from build123d import *

# Parameters (mm, degrees)
BOSS_EXTRUDE1_DEPTH      = 266.7
BOSS_EXTRUDE1_DEPTH_BACK = 266.7
SKETCH3_W                = 25.4
SKETCH3_H                = 25.4
SKETCH3_W_2              = 19.05
SKETCH3_H_2              = 19.05
SKETCH4_R                = 9.525
CUT_EXTRUDE1_DEPTH       = 25.4
SKETCH5_R                = 9.525
CUT_EXTRUDE2_DEPTH       = 3.175
F_10_CLEARANCE_HOLE1_D   = 4.9784
F_10_CLEARANCE_HOLE2_D   = 4.9784


with BuildPart() as part:
    # Sketch3 → Boss-Extrude1 (new, two sides: drawn at the far end of the back side and taken through both)
    with BuildSketch(Plane.XY.offset(-BOSS_EXTRUDE1_DEPTH_BACK)):
        Rectangle(SKETCH3_W, SKETCH3_H)
        Rectangle(SKETCH3_W_2, SKETCH3_H_2, mode=Mode.SUBTRACT)
    extrude(amount=BOSS_EXTRUDE1_DEPTH + BOSS_EXTRUDE1_DEPTH_BACK)

    # Sketch4 → Cut-Extrude1 (cut)
    with BuildSketch(Plane(origin=(0, 12.7, 0), x_dir=(1, 0, 0), z_dir=(0, 1, 0))):
        with Locations(Location((0, 212.725, 0), (0, 0, 180))):
            Circle(SKETCH4_R)
        Polygon((-12.7, 225.013453558), (-12.7, 266.7), (12.7, 266.7), (12.7, 252.73), (-3.69434815, 252.73), align=None)
    extrude(amount=-CUT_EXTRUDE1_DEPTH, mode=Mode.SUBTRACT)

    # Sketch5 → Cut-Extrude2 (cut)
    with BuildSketch(Plane.XZ.offset(12.7)):
        with Locations((-0.660548484, -179.870948658)):
            Circle(SKETCH5_R)
    extrude(amount=-CUT_EXTRUDE2_DEPTH, mode=Mode.SUBTRACT)

    # #10 Clearance Hole1 (through all)
    with Locations(Plane(origin=(12.7, 0, 0), x_dir=(0, 0, -1), z_dir=(1, 0, 0))):
        with Locations((212.725, 0)):
            Hole(F_10_CLEARANCE_HOLE1_D / 2)

    # #10 Clearance Hole2 (through all)
    with Locations(Plane(origin=(0, 12.7, 0), x_dir=(1, 0, 0), z_dir=(0, 1, 0))):
        with Locations((0, 153.95996007), (0, 237.806480142)):
            Hole(F_10_CLEARANCE_HOLE2_D / 2)


solid = part.part
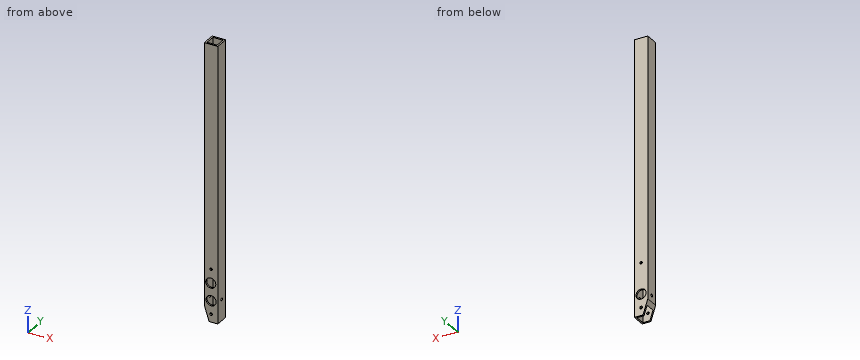
Source: CAD feature listing. Evaluate the final solid. Frame: model axes, mm. Coordinates: 2 decimals unless noted, no trailing zeros. Loops run counter-clockwise (first coordinate to the right, second up) from the corner with the lowest first, then second, coordinate; pieces in that order, holes last. Notation, with made-up numbers: M 30,75 L 86,75 A21 cw 86,104 Z; hole C 34.25,-34.5 d9. An arc over 180 degrees is marked long. Answer in a Markdown table with one row per item.
Q1. Section A-A on z = 157. Return the cut outline in (x, y) (3 decimals), plus the area to 3 significant figures.
Answers below:
| item | result |
|---|---|
| outline | M -12.7,-12.7 L 12.7,-12.7 L 12.7,12.7 L -12.7,12.7 Z; hole M -9.525,-9.525 L 9.525,-9.525 L 9.525,9.525 L -9.525,9.525 Z |
| area | 282 mm^2 |
Q2. Ray query, probe 1 along Z at (x, y) = (0, -11.45); probe 2 along Z at (x, y) = (0, 11.15); probe 3 along X at (y, z) = (7.25, 177) (3 decimals). Return the intervals inside material, ascending. Write a range as from..to.
Answers below:
| item | result |
|---|---|
| probe 1 | z = -252.73..-240.3, -235.32..-222.25, -203.2..-189.37, -170.37..-156.45, -151.47..266.7 |
| probe 2 | z = -252.73..-240.3, -235.32..-222.25, -203.2..-156.45, -151.47..266.7 |
| probe 3 | x = -12.7..-9.525, 9.525..12.7 |
Q3. First-contact query: pin 1 (4 mm diameter, centred on y = 0, z = -212.725, fed in from -X); pin 2 (15 mm diameter, centred on x = -0.66, z = -179.87, fed in from -Y) (3 decimals). Flat tips, straight axial feed; report the tip coordinate or a pass-through.
Answers below:
| item | result |
|---|---|
| pin 1 | passes through |
| pin 2 | stops at y = 9.525 |
